The listing builds one solid part. Answer for the finished solid, in the listing's coordinates (mm). Coordinates: 2 decimals unless noted, no trailing zeros. Order: outer loops, then holes, each group sorted by start corner. A loop starts at its lowest first (then second) coordinate and runs counter-clockwise, first axis right, second up. Notation, with made-up numbers: (24, -36) -> (81, -36) arc R22 cw to (81, 1) -> close; hole circle Ø5 at (73.5, 43.5). An arc over 180 degrees is marked (long way). One line per question, with ' | ' between items.
from build123d import *

# Parameters (mm, degrees)
CHAMFER1_SIZE = 0.16


with BuildPart() as part:
    # Sketch1 → Revolve1 (revolve)
    with BuildSketch(Plane.XY, mode=Mode.PRIVATE) as revolve1_sk:
        with BuildLine():
            Line((-4.206651636, 0), (-1.6, 0))
            Line((-1.6, 0), (-1.6, -5))
            Line((-1.6, -5), (-4.206651636, -5))
            ThreePointArc((-4.206651636, -5), (-4.619513048, -4.782038037), (-4.672422125, -4.318181818))
            ThreePointArc((-4.672422125, -4.318181818), (-4.330127019, -2.5), (-4.672422125, -0.681818182))
            ThreePointArc((-4.672422125, -0.681818182), (-4.619513048, -0.217961963), (-4.206651636, 0))
        make_face()
    revolve(revolve1_sk.sketch.rotate(Axis((0, 0, 0), (0, -1, 0)), 270), axis=Axis((0, 0, 0), (0, -1, 0)))

    # Chamfer1
    chamfer1_edges = [part.edges().sort_by_distance(p)[0] for p in [
        (0, -5, -1.6),
    ]]
    chamfer(chamfer1_edges, length=CHAMFER1_SIZE)


solid = part.part
Item 1: Section D-D, the plane y = -2.3 is taken. Give the vertices of the cut face in (x, z), plus the area to 3 significant figures.
Computed values:
outline: circle Ø8.67 at (0, 0); hole circle Ø3.2 at (0, 0) | area: 51.0 mm^2
Item 2: Each of these flat-tipped pins is pushed along its axis until it touches: pin 1 Ø2 at (x, y) = (3, -0.5) entering from +Z; pin 2 Ø1.5 at (y, z) = (-3.5, -0.5) entering from +X; pin 3 Ø1 at (x, y) = (-2.5, -1.5) entering from +Z. Where does it stop, or does it pass through?
Computed values:
pin 1: stops at z = 4.26 | pin 2: stops at x = 4.63 | pin 3: stops at z = 3.98
Item 3: Section B-B, the plane z = 0 is taken. Give the vertices of the cut face in (x, y).
Computed values:
outline: (-4.67, -4.32) arc R0.5 ccw to (-4.21, -5) -> (-1.76, -5) -> (-1.6, -4.84) -> (-1.6, 0) -> (-4.21, 0) arc R0.5 ccw to (-4.67, -0.68) arc R5 cw to start; (1.6, -4.84) -> (1.76, -5) -> (4.21, -5) arc R0.5 ccw to (4.67, -4.32) arc R5 cw to (4.67, -0.68) arc R0.5 ccw to (4.21, 0) -> (1.6, 0) -> close
Item 4: Determine the mould class of faces 1 (the face through (2, -5, 0)), 2 (the face through (0.97, -2.45, -1.27)) for opening direction X: pulls with the +X half, pulls with the -X half, needs draft (parallel to the pull), parting line crosses it, or undercut.
Computed values:
face 1: needs draft | face 2: undercut
Item 5: Find the intervals of material crossed by L1, parallel to X at y = -1.5, z = 0; L2, parallel to X at y = -1.3, z = 0; L3, parallel to Y at x = 2.75, z = -3.25, in increasing order.
Computed values:
L1: x = -4.43 to -1.6, 1.6 to 4.43 | L2: x = -4.48 to -1.6, 1.6 to 4.48 | L3: y = -5 to 0
Item 6: Section C-C, the plane y = -3.1 is taken. Give the vertices of the cut face in (x, z), plus the area to 3 significant figures.
Computed values:
outline: circle Ø8.73 at (0, 0); hole circle Ø3.2 at (0, 0) | area: 51.8 mm^2
Item 7: Section A-A, the plane x = 0 is taken. Give the vertices of the cut face in (y, z).
Computed values:
outline: (-5, -4.21) arc R0.5 ccw to (-4.32, -4.67) arc R5 cw to (-0.68, -4.67) arc R0.5 ccw to (0, -4.21) -> (0, -1.6) -> (-4.84, -1.6) -> (-5, -1.76) -> close; (-5, 1.76) -> (-4.84, 1.6) -> (0, 1.6) -> (0, 4.21) arc R0.5 ccw to (-0.68, 4.67) arc R5 cw to (-4.32, 4.67) arc R0.5 ccw to (-5, 4.21) -> close
